from build123d import *

# Parameters (mm, degrees)
CROQUIS1_R              = 1.5
SALIENTE_EXTRUIR1_DEPTH = 3
CROQUIS3_W              = 22
CROQUIS3_H              = 37
SALIENTE_EXTRUIR2_DEPTH = 13
CORTAR_EXTRUIR1_START   = -37
CORTAR_EXTRUIR1_DEPTH   = 37
SALIENTE_EXTRUIR4_DEPTH = 6
CROQUIS7_W              = 3.002058729
CROQUIS7_H              = 21
CORTAR_EXTRUIR2_DEPTH   = 22.000001
CROQUIS8_W              = 3
CROQUIS8_H              = 43
SALIENTE_EXTRUIR5_DEPTH = 25


with BuildPart() as part:
    # Croquis1 → Saliente-Extruir1 (new body)
    with BuildSketch(Plane.XY):
        with BuildLine():
            Line((-4.197309417, 33.461883408), (-52.197309417, 33.461883408))
            ThreePointArc((-52.197309417, 33.461883408), (-55.025736542, 32.290310533), (-56.197309417, 29.461883408))
            Line((-56.197309417, 29.461883408), (-56.197309417, 24.961883408))
            Line((-56.197309417, 24.961883408), (-49.197309417, 24.961883408))
            Line((-49.197309417, 24.961883408), (-49.197309417, 4.961883408))
            Line((-49.197309417, 4.961883408), (-56.197309417, 4.961883408))
            Line((-56.197309417, 4.961883408), (-56.197309417, 0.461883408))
            ThreePointArc((-56.197309417, 0.461883408), (-55.099110766, -2.293519818), (-52.406664651, -3.538116592))
            Line((-52.406664651, -3.538116592), (-4.197309417, -3.538116592))
            Line((-4.197309417, -3.538116592), (-4.197309417, 7.961883408))
            Line((-4.197309417, 7.961883408), (-10.197309417, 7.961883408))
            Line((-10.197309417, 7.961883408), (-10.197309417, 21.961883408))
            Line((-10.197309417, 21.961883408), (-4.197309417, 21.961883408))
            Line((-4.197309417, 21.961883408), (-4.197309417, 33.461883408))
        make_face()
        with Locations((-52.19152813, 0.461883408)):
            Circle(CROQUIS1_R, mode=Mode.SUBTRACT)
        with Locations((-8.197309417, 0.461883408)):
            Circle(CROQUIS1_R, mode=Mode.SUBTRACT)
        with Locations((-52.197309417, 29.461883408)):
            Circle(CROQUIS1_R, mode=Mode.SUBTRACT)
        with Locations((-8.197309417, 29.461883408)):
            Circle(CROQUIS1_R, mode=Mode.SUBTRACT)
    extrude(amount=SALIENTE_EXTRUIR1_DEPTH)

    # Croquis3 → Saliente-Extruir2 (add)
    with BuildSketch(Plane.XY.offset(3)):
        with Locations((-38.197309417, 14.961883408)):
            Rectangle(CROQUIS3_W, CROQUIS3_H)
    extrude(amount=SALIENTE_EXTRUIR2_DEPTH)

    # Croquis4 → Cortar-Extruir1 (cut)
    with BuildSketch(Plane.XZ.offset(3.538116592).offset(CORTAR_EXTRUIR1_START)):
        Polygon((-27.197309417, 16), (-27.197309417, 6.002058729), (-49.197309417, 16), align=None)
    extrude(amount=CORTAR_EXTRUIR1_DEPTH, mode=Mode.SUBTRACT)

    # Croquis6 → Saliente-Extruir4 (add)
    with BuildSketch(Plane(origin=(0, 33.461883408, 0), x_dir=(1, 0, 0), z_dir=(0, 1, 0))):
        Polygon((-27.197309417, -6.002058729), (-49.197309417, -16), (-49.197309417, 0), (-27.197309417, 0), align=None)
    extrude(amount=SALIENTE_EXTRUIR4_DEPTH)

    # Croquis7 → Cortar-Extruir2 (cut)
    with BuildSketch(Plane(origin=(-27.197309417, 0, 0), x_dir=(0, 0, -1), z_dir=(1, 0, 0))):
        with Locations((-4.501029365, 25.961883408)):
            Rectangle(CROQUIS7_W, CROQUIS7_H)
    extrude(amount=-CORTAR_EXTRUIR2_DEPTH, mode=Mode.SUBTRACT)

    # Croquis8 → Saliente-Extruir5 (add)
    with BuildSketch(Plane(origin=(-2.394740987, 0, -5.269515022), x_dir=(0.9103985682863143, 0, -0.4137323372208525), z_dir=(0.4137323372208525, 0, 0.9103985682863143))):
        with Locations((-28.743637341, 17.961883408)):
            Rectangle(CROQUIS8_W, CROQUIS8_H)
    extrude(amount=SALIENTE_EXTRUIR5_DEPTH)


solid = part.part
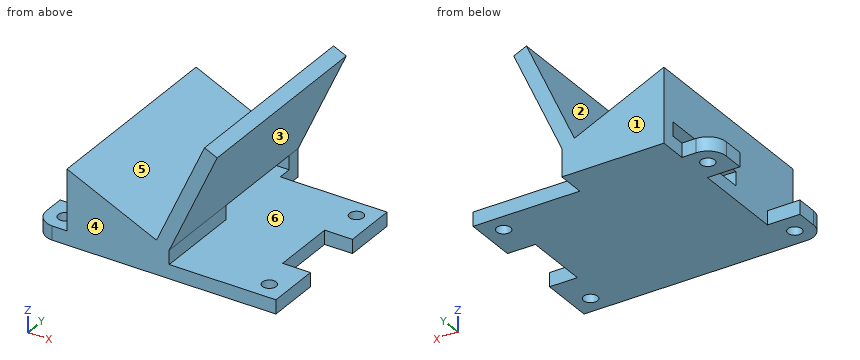
The listing builds one solid part. Answer for the finished solid, in the listing's coordinates (mm). Face numbers are marked on the shaded views. A direction names the side the tool comes from. Coordinates: 2 decimals unless noted, no trailing zeros. Write each loop counter-clockwise with the first axis right and the second up, starting at its lowest first coordinate (ties: lowest second). Pieces come first, ordered by that corner, then holes. Notation, with made-up numbers: (-17.75, 59.5) - (1.25, 59.5) arc R26 cw to (1.25, 81.5) - close; hole circle Ø5 at (51.5, -29.75). An arc over 180 degrees is marked (long way). Return JSON: item names as keys, results as strings.
1. Consider line 1 along Z through (x, y) = (-51, 2); line 2 along Z through (x, y) = (-33, 26); line 3 along Z through (x, y) = (-26, 14). Determine where each line is inside the solid, lowest interval first.
Final values:
{"line 1": "0 to 3", "line 2": "0 to 3, 6 to 8.64", "line 3": "0 to 3, 8.64 to 15.89"}
2. The part is cut by section C-C on x = -32. Determine the outline of the cut face in (y, z), then the cut area to 3 significant figures.
Final values:
{"outline": "(-3.54, 0) - (39.46, 0) - (39.46, 8.18) - (-3.54, 8.18) - close; hole (15.46, 3) - (36.46, 3) - (36.46, 6) - (15.46, 6) - close", "area": "289 mm^2"}
3. Which of the six approach directions +Z, -Z, +X, -X, +Y, -Y give full straight-line access (tool end or side, diameter ignored) to the marked faces 1, 2 and 3?
Final values:
{"face 1": "+Z, -Z, +X, -X, +Y", "face 2": "+Z, +Y, -Y", "face 3": "+X, +Y, -Y"}
4. Each of these flat-tipped pins is pushed along its axis until it touches: pin 1 Ø6 at (x, z) = (-21, 17) entering from +Y; pin 2 Ø2.5 at (y, z) = (18, 2) entering from +X; pin 3 Ø12 at (y, z) = (23, 11.5) entering from -X; pin 4 Ø1.8 at (y, z) = (36.5, 1.5) entering from +X. Where does it stop, or does it pass through?
Final values:
{"pin 1": "y = 39.46", "pin 2": "x = -10.2", "pin 3": "x = -49.2", "pin 4": "x = -27.2"}
5. The part is cut by section D-D on y = 6. Determine the outline of the cut face in (x, z).
Final values:
{"outline": "(-49.2, 0) - (-4.2, 0) - (-4.2, 3) - (-27.2, 3) - (-27.2, 6) - (-16.85, 28.76) - (-19.59, 30) - (-29.93, 7.24) - (-49.2, 16) - close"}
6. For a pull along Y with two mould halves and no side action, classify the marked faces 4, 5 and 6 as +Y half, -Y half, draft (parallel to the pull), parting line (faces both ways), or undercut.
Final values:
{"face 4": "-Y half", "face 5": "draft", "face 6": "undercut"}
7. The part is cut by section A-A on y = 26.5. Determine the outline of the cut face in (x, z).
Final values:
{"outline": "(-56.2, 0) - (-4.2, 0) - (-4.2, 3) - (-56.2, 3) - close; (-49.2, 6) - (-27.2, 6) - (-16.85, 28.76) - (-19.59, 30) - (-29.93, 7.24) - (-49.2, 16) - close"}
8. The part is cut by section B-B on z = 10. Determine the outline of the cut face in (x, y), then the cut area to 3 significant figures.
Final values:
{"outline": "(-49.2, -3.54) - (-35.99, -3.54) - (-35.99, 39.46) - (-49.2, 39.46) - close; (-28.68, -3.54) - (-25.38, -3.54) - (-25.38, 39.46) - (-28.68, 39.46) - close", "area": "709 mm^2"}
